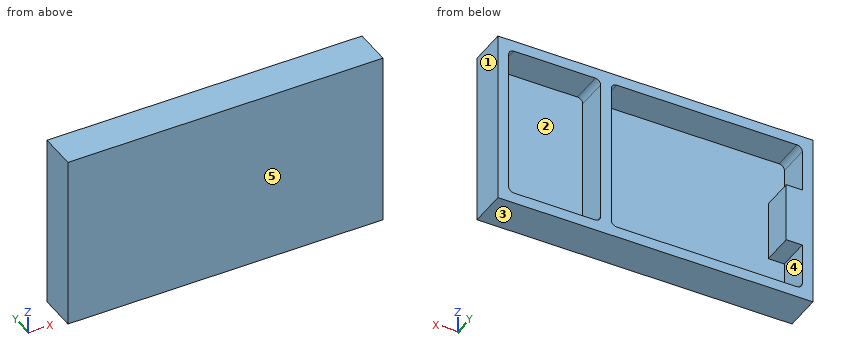
```python
from build123d import *

# Parameters (mm, degrees)
SKETCH11_W     = 187.05178758
SKETCH11_H     = 103.91050065
EXTRUDE3_DEPTH = 19.05
SKETCH12_W     = 187.05178758
SKETCH12_H     = 103.91050065
EXTRUDE4_DEPTH = 3.175
SKETCH15_W     = 35.329261405
SKETCH15_H     = 19.05
EXTRUDE6_DEPTH = 9.525


with BuildPart() as part:
    # Sketch11 → Extrude3 (new body)
    with BuildSketch(Plane(origin=(0, 0, 0), x_dir=(1, 0, 0), z_dir=(0, 1, 0))):
        with Locations((93.52589379, 51.955250325)):
            Rectangle(SKETCH11_W, SKETCH11_H)
        with BuildLine():
            Line((9.525, 6.35), (116.541319734, 6.35))
            ThreePointArc((116.541319734, 6.35), (118.786383764, 7.27993597), (119.716319734, 9.525))
            Line((119.716319734, 9.525), (119.716319734, 94.38550065))
            ThreePointArc((119.716319734, 94.38550065), (118.786383764, 96.63056468), (116.541319734, 97.56050065))
            Line((116.541319734, 97.56050065), (9.525, 97.56050065))
            ThreePointArc((9.525, 97.56050065), (7.27993597, 96.63056468), (6.35, 94.38550065))
            Line((6.35, 94.38550065), (6.35, 9.525))
            ThreePointArc((6.35, 9.525), (7.27993597, 7.27993597), (9.525, 6.35))
        make_face(mode=Mode.SUBTRACT)
        with BuildLine():
            Line((180.70178758, 9.525), (180.70178758, 94.38550065))
            ThreePointArc((180.70178758, 94.38550065), (179.77185161, 96.63056468), (177.52678758, 97.56050065))
            Line((177.52678758, 97.56050065), (129.241319734, 97.56050065))
            ThreePointArc((129.241319734, 97.56050065), (126.996255703, 96.63056468), (126.066319734, 94.38550065))
            Line((126.066319734, 94.38550065), (126.066319734, 9.525))
            ThreePointArc((126.066319734, 9.525), (126.996255703, 7.27993597), (129.241319734, 6.35))
            Line((129.241319734, 6.35), (177.52678758, 6.35))
            ThreePointArc((177.52678758, 6.35), (179.77185161, 7.27993597), (180.70178758, 9.525))
        make_face(mode=Mode.SUBTRACT)
    extrude(amount=EXTRUDE3_DEPTH)

    # Sketch12 → Extrude4 (add)
    with BuildSketch(Plane(origin=(0, 0, 0), x_dir=(1, 0, 0), z_dir=(0, 1, 0))):
        with Locations((93.52589379, 51.955250325)):
            Rectangle(SKETCH12_W, SKETCH12_H)
    extrude(amount=-EXTRUDE4_DEPTH)

    # Sketch15 → Extrude6 (add)
    with BuildSketch(Plane(origin=(6.35, 0, 0), x_dir=(0, 0, -1), z_dir=(1, 0, 0))):
        with Locations((51.955250324, 9.525)):
            Rectangle(SKETCH15_W, SKETCH15_H)
    extrude(amount=EXTRUDE6_DEPTH)


solid = part.part
```
Input: part model. Units: mm. Frame: model coordinates. Face numbers are marked on the shaded views. A direction names the side the tool comes from. Coordinates: 2 decimals unless noted, no trailing zeros. Write each loop counter-clockwise with the first axis right and the second up, starting at its lowest first coordinate (ties: lowest second). Pieces come first, ordered by that corner, then holes.
1) Pin query (flat end, axial travel): pin 1 Ø8 at (x, z) = (141.5, -16.5) entering from +Y. Return the tip coordinate at first contact, or that it passes through.
2) Section D-D on z = -59. Output: boundary loops of the cut face in (x, y) (3 decimals), and give its area (3 significant figures).
3) Section C-C on y = 3.25. State how many separate pieces and enclosed holes the cut face has, and give its area (3 significant figures).
4) Set-up query: the marked faces 4 and 5. Return all of +Z, -Z, +X, -X, +Y, -Y with unobstructed straight access to the full face (end or side cutting, diameter ignored); none if empty.
5) Mould query, pull axis Z, two halves, no side actions, for the marked faces 1, 2 and 3. Classes: pulls with the +Z half, pulls with the -Z half, needs draft (parallel to the pull), parting line crosses it, or undercut.
6) Section A-A on z = -32.5. Output: boundary loops of the cut face in (x, y) (3 decimals).
7) Material intervals for line 1 along X through (y, z) = (16.5, -81); line 2 along X through (y, z) = (8.5, -48.5) (3 decimals); line 3 along Z through (x, y) = (83.5, 17.5), sorted ascending.
Check result:
1. pin 1: stops at y = 0
2. outline: (0, -3.175) - (187.052, -3.175) - (187.052, 19.05) - (180.702, 19.05) - (180.702, 0) - (126.066, 0) - (126.066, 19.05) - (119.716, 19.05) - (119.716, 0) - (15.875, 0) - (15.875, 19.05) - (0, 19.05) - close
2. area: 1,140 mm2
3. separate pieces: 1
3. enclosed holes: 2
3. area: 4,470 mm2
4. face 4: +Y
4. face 5: +Z, -Z, +X, -X, -Y
5. face 1: needs draft
5. face 2: undercut
5. face 3: pulls with the -Z half
6. outline: (0, -3.175) - (187.052, -3.175) - (187.052, 19.05) - (180.702, 19.05) - (180.702, 0) - (126.066, 0) - (126.066, 19.05) - (119.716, 19.05) - (119.716, 0) - (6.35, 0) - (6.35, 19.05) - (0, 19.05) - close
7. line 1: x = 0 to 6.35, 119.72 to 126.07, 180.7 to 187.05
7. line 2: x = 0 to 15.875, 119.716 to 126.066, 180.702 to 187.052
7. line 3: z = -103.91 to -97.56, -6.35 to 0
